Check sheet for the modelled part. Datum: model origin and axes. Units: mm. A direction names the side the tool comes from. Coordinates: 2 decimals unless noted, no trailing zeros. Loops run counter-clockwise (first coordinate to the right, second up) from the corner with the lowest first, then second, coordinate; pieces in that order, holes last. Notation, with made-up numbers: (36.25, 11.5) - (50.25, 11.5) arc R22 ccw to (50.25, 22.5) - close; hole circle Ø9 at (14, 43). An arc over 180 degrees is marked (long way). Use a Markdown table: item, result. Add a question column.
1) Sectioned sample at B-B, the plane z = -57.15. Enter the section's corners in (x, y), then the cut area to 3 significant figures.
2) Go/stop test with flat-tipped pins: P1, Ø1.5, axis at y = 3, z = -16.5, coming from the +X side; P2, Ø3, axis at y = 2.5, z = -42.5, coming from the +X side; P3, Ø2, axis at x = -4.5, y = 2, coming from the +Z side. Record where each tip stops, or that it passes through.
3) Tool access check on faces 4 (the flat face through (-25.4, 3, -59)), 5 (the cylindrical face through (11.469, 3.131, 10.976)). Record the directions out of +Z, -Z, +X, -X, +Y, -Y that give a thin tool (end or side, any length) a straight path to the whole face; none if there is none.
4) Sectioned sample at A-A, the plane y = 4.25. State how many separate pieces and enclosed holes the cut face has, then the cut area to 3 significant figures.
5) Draft check along Z on faces 1 (the cylindrical face through (-54.666, 3.131, -35.539)), 2 (the flat face through (-57.15, 3, -59)), 3 (the cylindrical face through (-51.14, 3.22, -55.6)). Enter one of: pulls with the +Z half, pulls with the -Z half, needs draft (parallel to the pull), parting line crosses it, or undercut.
6) Thickness scan on line 1 (X direction, y = 2.5, z = -57.15); line 2 (Z direction, x = -31.75, y = 1.5); line 3 (Z direction, x = 0, y = 5). Record the ranges inside material, lowest first.
7) Sectioned sample at D-D, the plane z = -2. Enter the section's corners in (x, y).
8) Sectioned sample at C-C, the plane x = -31.75. Enter the section's corners in (y, z).
Autodesk Inventor part; units mm, degrees
ref_plane "YZ Plane" through (0, 0, 0) normal (1, 0, 0) x (0, 1, 0)
ref_plane "XZ Plane" through (0, 0, 0) normal (0, 1, 0) x (-1, 0, 0)
ref_plane "XY Plane" through (0, 0, 0) normal (0, 0, 1) x (1, 0, 0)
sketch "Sketch1" plane through (0, 0, 0) normal (0, 1, 0) x (-1, 0, 0)
  circle A0 centre (0, 0) radius 4.7625
  line L0 (0, -228.6) -> (0, 0) construction
  line L1 (15.875, -228.6) -> (0, -228.6) construction
  circle A1 centre (15.875, -228.6) radius 7.9375
  line L2 (25.4, -47.8506) -> (25.4, -212.725)
  line L3 (57.15, -47.8506) -> (57.15, -212.725)
  line L4 (25.4, -212.725) -> (15.875, -212.725)
  arc A2 (15.875, -212.725) -> (15.875, -244.475) centre (15.875, -228.6) ccw
  line L5 (15.875, -244.475) -> (25.4, -244.475)
  arc A3 (25.4, -244.475) -> (57.15, -212.725) centre (25.4, -212.725) ccw
  line L6 (57.15, -130.2878) -> (25.4, -130.2878) construction
  arc A4 (11.2253, 11.2253) -> (-11.2253, -11.2253) centre (0, 0) ccw
  line L7 (-11.2253, -11.2253) -> (25.4, -47.8506)
  arc A5 (57.15, -47.8506) -> (47.8506, -25.4) centre (25.4, -47.8506) ccw
  line L8 (47.8506, -25.4) -> (11.2253, 11.2253)
  line L9 (41.275, -130.2878) -> (41.275, -240.2213) construction
  line L10 (41.275, -130.2878) -> (41.275, -18.8244) construction
  dimension "d0" = 9.525
  dimension "d2" = 228.6
  dimension "d7" = 15.875
  dimension "d17" = 31.75
  dimension "d18" = 45
  dimension "d19" = 25.4
  dimension "d20" = 25.4
extrude "Extrusion1" add sketch "Sketch1" along normal blind 6.35
sketch "Sketch2" plane through (0, 6.35, 0) normal (0, 1, 0) x (1, 0, 0)
  line L0 (-69.0057, 276.0917) -> (22.485, 276.0917)
  line L1 (22.485, 276.0917) -> (22.485, 69.85)
  line L2 (22.485, 69.85) -> (-69.0057, 69.85)
  line L3 (-69.0057, 69.85) -> (-69.0057, 276.0917)
  point P0 (0, 0)
  dimension "d21" = 69.85
extrude "Extrusion2" cut sketch "Sketch2" against normal through all
sketch "Sketch3" plane through (0, 6.35, 0) normal (0, 1, 0) x (1, 0, 0)
  line L0 (-25.4, 47.8506) -> (-25.4, 69.85) construction
  line L1 (-25.4, 47.8506) -> (-25.4, 69.85) construction
  line L2 (-25.4, 57.15) -> (-57.15, 57.15) construction
  line L3 (-25.4, 69.85) -> (-57.15, 69.85) construction
  line L4 (-41.275, 69.85) -> (-41.275, 57.15) construction
  circle A0 centre (-50.8, 57.15) radius 1.5875
  circle A1 centre (-31.75, 57.15) radius 1.5875
  point P0 (0, 0)
  dimension "d24" = 12.7
  dimension "d26" = 3.175
  dimension "d27" = 19.05
extrude "Extrusion3" cut sketch "Sketch3" against normal through all
properties part number "Cross Arms"
Solved:
| question | item | result |
|---|---|---|
| 1 | outline | (-57.15, 0) - (-52.39, 0) - (-52.39, 6.35) - (-57.15, 6.35) - close; (-49.21, 0) - (-33.34, 0) - (-33.34, 6.35) - (-49.21, 6.35) - close; (-30.16, 0) - (-25.4, 0) - (-25.4, 6.35) - (-30.16, 6.35) - close |
| 1 | area | 161 mm2 |
| 2 | P1 | stops at x = 6.7 |
| 2 | P2 | stops at x = -18.55 |
| 2 | P3 | stops at z = 15.48 |
| 3 | face 4 | -Z, +X, +Y, -Y |
| 3 | face 5 | +Y, -Y |
| 4 | separate pieces | 1 |
| 4 | enclosed holes | 3 |
| 4 | area | 3,050 mm2 |
| 5 | face 1 | pulls with the +Z half |
| 5 | face 2 | needs draft |
| 5 | face 3 | undercut |
| 6 | line 1 | x = -57.15 to -52.39, -49.21 to -33.34, -30.16 to -25.4 |
| 6 | line 2 | z = -69.85 to -58.74, -55.56 to -9.3 |
| 6 | line 3 | z = -22.45 to -4.76, 4.76 to 15.87 |
| 7 | outline | (-24.45, 0) - (-4.32, 0) - (-4.32, 6.35) - (-24.45, 6.35) - close; (4.32, 0) - (15.75, 0) - (15.75, 6.35) - (4.32, 6.35) - close |
| 8 | outline | (0, -69.85) - (6.35, -69.85) - (6.35, -58.74) - (0, -58.74) - close; (0, -55.56) - (6.35, -55.56) - (6.35, -9.3) - (0, -9.3) - close |
